Drawing for the job (mm, zero at the part's lowest x, y, z). A direction names the side the tool comes from. Round coordinates to 2 decimals unless told otherwise and drop trailing zeros. Write each loop counter-clockwise with the first axis right and the second up, starting at its lowest first coordinate (ties: lowest second). Pieces come first, ordered by that corner, then holes. Notation, with made-up numbers: (14.25, 48) -> (32.25, 48) arc R25 cw to (32.25, 83) -> close; hole circle Ø5 at (-19, 54.25). An arc over 180 degrees is marked (long way). Answer in a Markdown table with one row per item. Add a question column.
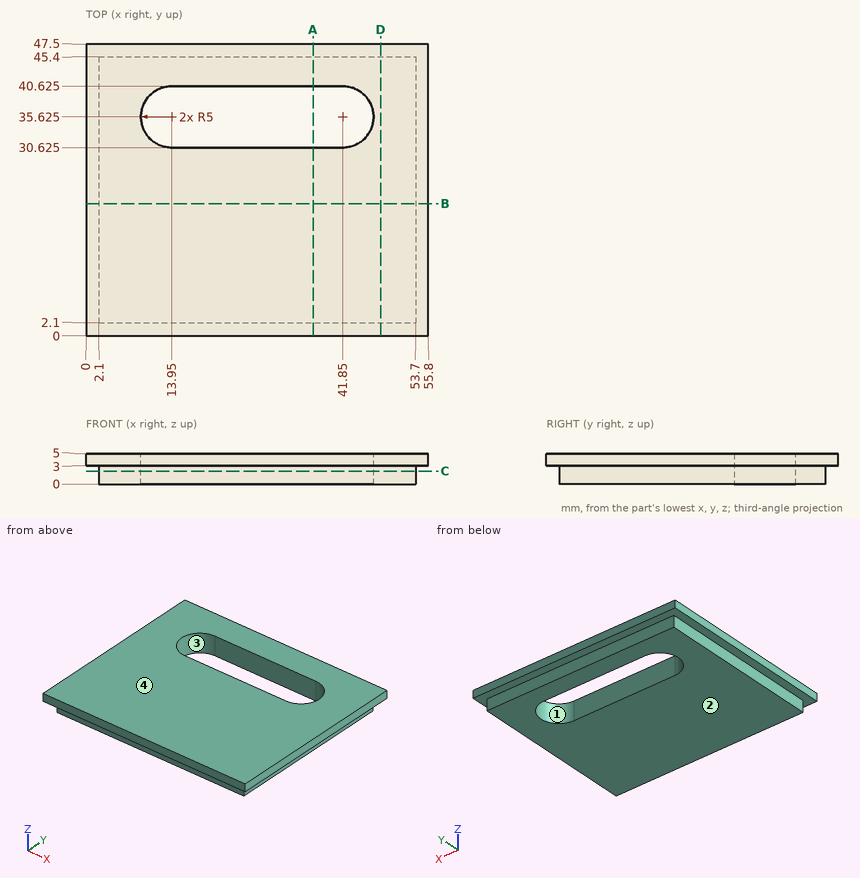
(1) Saw through at A-A (x = 37). List the corners of the cut face in (y, z) (3 decimals).
(2) Saw through at D-D (x = 48). List the corners of the cut face in (y, z).
(3) Probe line 1 along Y through (x, z) = (39, 3.95) (3 decimals); line 2 along Y through (x, z) = (26, 1.6) (3 decimals); line 3 along Y through (x, z) = (4, 0.65). List the from-to ranges inside material, lowest first.
(4) Mould opens along X. For the marked faces 1 and 2 say: pulls with the +X half, pulls with the -X half, needs draft (parallel to the pull), parting line crosses it, or undercut.
(5) Which spindle directions (+Z, -Z, +X, -X, +Y, -Y) get a long thin tool onto all of the face, cutting with end or side? Do the marked faces 3 and 4. Say none if no direction does.
(6) Saw through at B-B (y = 21.5). List the corners of the cut face in (x, z), plus the area to 3 significant figures.
(7) Saw through at C-C (z = 2.15). List the corners of the cut face in (x, y) (3 decimals).
(8) Drop flat-ended pins along their axis: P1, Ø0.9, axis at y = 18, z = 1, coming from the +X side; P2, Ø1, axis at x = 48, z = 1.5, coming from the -Y side; P3, Ø0.9, axis at x = 17.5, z = 2, coming from the +Y side. Give the stop position or say it passes through.
Answer sheet:
| question | item | result |
|---|---|---|
| 1 | outline | (0, 3) -> (2.1, 3) -> (2.1, 0) -> (30.625, 0) -> (30.625, 5) -> (0, 5) -> close; (40.625, 0) -> (45.4, 0) -> (45.4, 3) -> (47.5, 3) -> (47.5, 5) -> (40.625, 5) -> close |
| 2 | outline | (0, 3) -> (2.1, 3) -> (2.1, 0) -> (45.4, 0) -> (45.4, 3) -> (47.5, 3) -> (47.5, 5) -> (0, 5) -> close |
| 3 | line 1 | y = 0 to 30.625, 40.625 to 47.5 |
| 3 | line 2 | y = 2.1 to 30.625, 40.625 to 45.4 |
| 3 | line 3 | y = 2.1 to 45.4 |
| 4 | face 1 | undercut |
| 4 | face 2 | needs draft |
| 5 | face 3 | +Z, -Z |
| 5 | face 4 | +Z, +X, -X, +Y, -Y |
| 6 | outline | (0, 3) -> (2.1, 3) -> (2.1, 0) -> (53.7, 0) -> (53.7, 3) -> (55.8, 3) -> (55.8, 5) -> (0, 5) -> close |
| 6 | area | 266 mm² |
| 7 | outline | (2.1, 2.1) -> (53.7, 2.1) -> (53.7, 45.4) -> (2.1, 45.4) -> close; hole (13.95, 30.625) -> (41.85, 30.625) arc R5 ccw to (41.85, 40.625) -> (13.95, 40.625) arc R5 ccw to start |
| 8 | P1 | stops at x = 53.7 |
| 8 | P2 | stops at y = 2.1 |
| 8 | P3 | stops at y = 45.4 |
